from build123d import *

# Parameters (mm, degrees)
SKETCH1_R           = 3.175
BOSS_EXTRUDE2_DEPTH = 30
CHAMFER1_SIZE       = 0.25
CHAMFER2_SIZE       = 0.25
SKETCH10_R          = 2.632684592
CUT_EXTRUDE2_DEPTH  = 34
FILLET2_R           = 0.25
FILLET3_R           = 0.25


with BuildPart() as part:
    # Sketch1 → Boss-Extrude2 (new body)
    with BuildSketch(Plane(origin=(0, 0, 0), x_dir=(1, 0, 0), z_dir=(0, 1, 0))):
        Circle(SKETCH1_R)
    extrude(amount=BOSS_EXTRUDE2_DEPTH)

    # Chamfer1
    chamfer1_edges = [part.edges().sort_by_distance(p)[0] for p in [
        (-3.175, 30, 0),
    ]]
    chamfer(chamfer1_edges, length=CHAMFER1_SIZE)

    # Chamfer2
    chamfer2_edges = [part.edges().sort_by_distance(p)[0] for p in [
        (-3.175, 0, 0),
    ]]
    chamfer(chamfer2_edges, length=CHAMFER2_SIZE)

    # Sketch10 → Cut-Extrude2 (cut)
    with BuildSketch(Plane(origin=(0, 0, 0), x_dir=(1, 0, 0), z_dir=(0, 1, 0))):
        Circle(SKETCH10_R)
    extrude(amount=CUT_EXTRUDE2_DEPTH, mode=Mode.SUBTRACT)

    # Fillet2
    fillet2_edges = [part.edges().sort_by_distance(p)[0] for p in [
        (-2.925, 30, 0),
    ]]
    fillet(fillet2_edges, radius=FILLET2_R)

    # Fillet3
    fillet3_edges = [part.edges().sort_by_distance(p)[0] for p in [
        (-2.925, 0, 0),
    ]]
    fillet(fillet3_edges, radius=FILLET3_R)


solid = part.part
CAD build for the part. Positions are in the model's coordinates, mm. Round coordinates to 2 decimals unless told otherwise and drop trailing zeros. Write each loop counter-clockwise with the first axis right and the second up, starting at its lowest first coordinate (ties: lowest second). Pieces come first, ordered by that corner, then holes. Notation, with made-up numbers: (27.5, 7.25) -> (60.5, 7.25) arc R32 ccw to (60.5, 35.25) -> close; hole circle Ø8 at (62, 25.25). An arc over 180 degrees is marked (long way). Answer as a JSON object with one key per item and string values.
(1) Probe probe 1 along X at (y, z) = (21.25, 0) (3 decimals); probe 2 along X at (y, z) = (16, -1.25). List the from-to ranges inside material, lowest first. Write a range as [from, to].
Reported:
{"probe 1": "x = [-3.175, -2.633], [2.633, 3.175]", "probe 2": "x = [-2.92, -2.32], [2.32, 2.92]"}
(2) Two-plate mould, pull along X, no slides. Class faces 1 (the face through (1.415, 14.79, -2.22)), 2 (the face through (-0.69, 14.79, 3.1)): +X half, -X half, draft (parallel to the pull), parting line (faces both ways), or undercut.
Reported:
{"face 1": "undercut", "face 2": "parting line"}
(3) Band-saw the part on A-A, the plane x = 0. List the corners of the cut face in (y, z) (3 decimals), then the cut area to 3 significant figures.
Reported:
{"outline": "(0, -2.821) arc R0.25 ccw to (0.073, -2.998) -> (0.25, -3.175) -> (29.75, -3.175) -> (29.927, -2.998) arc R0.25 ccw to (30, -2.821) -> (30, -2.633) -> (0, -2.633) -> close; (0, 2.633) -> (30, 2.633) -> (30, 2.821) arc R0.25 ccw to (29.927, 2.998) -> (29.75, 3.175) -> (0.25, 3.175) -> (0.073, 2.998) arc R0.25 ccw to (0, 2.821) -> close", "area": "32.4 mm^2"}
(4) Pin check, flat tips, straight feed: P1, Ø1.5, axis at y = 16, z = -1.5, coming from the +X side; P2, Ø2, axis at x = 1.5, z = -0.5, coming from the -Y side; P3, Ø3, axis at x = -2, y = 26, coming from the -Z side. Stop position of each tip, or through.
Reported:
{"P1": "stops at x = 3.09", "P2": "passes through", "P3": "stops at z = -3.14"}
(5) Band-saw the part on B-B, the plane y = 28.25. List the corners of the cut face in (x, z) (3 decimals), then the cut area to 3 significant figures.
Reported:
{"outline": "circle Ø6.35 at (0, 0); hole circle Ø5.265 at (0, 0)", "area": "9.89 mm^2"}
